Source: CAD feature listing. Evaluate the final solid. Frame: model axes, mm. Give positions to 0.01 mm unless a question says otherwise; leave off trailing zeros. Order: outer loops, then holes, each group sorted by start corner. A loop starts at its lowest first (then second) coordinate and runs counter-clockwise, first axis right, second up. Notation, with made-up numbers: (-1.75, 64) -> (15.25, 64) arc R23 ccw to (15.25, 102) -> close; hole circle Ø10 at (86, 57.5). An arc over 180 degrees is marked (long way). Use CSV: the item, a comma, the result in double quotes.
Autodesk Fusion 360 part; units mm, degrees
sketch "スケッチ1" plane through (0, 0, 0) normal (0, 1, 0) x (1, 0, 0)
  line L0 (30, 20) -> (-30, 20)
  line L1 (-30, 20) -> (-30, -20)
  line L2 (-30, -20) -> (30, -20)
  line L3 (30, -20) -> (30, 20)
  line L4 (30, 20) -> (-30, -20) construction
  line L5 (-30, 20) -> (30, -20) construction
  line L6 (-20, 0) -> (20, 0)
  dimension "d1" = 60
  dimension "d2" = 40
  dimension "d3" = 40
extrude "押し出し1" add sketch "スケッチ1" along normal blind 10
hole "穴1" at (-20, 0, 0) at (20, 0, 0) direction (0, 1, 0) diameter 3 depth 12 tip angle 118
thread "ねじ1"
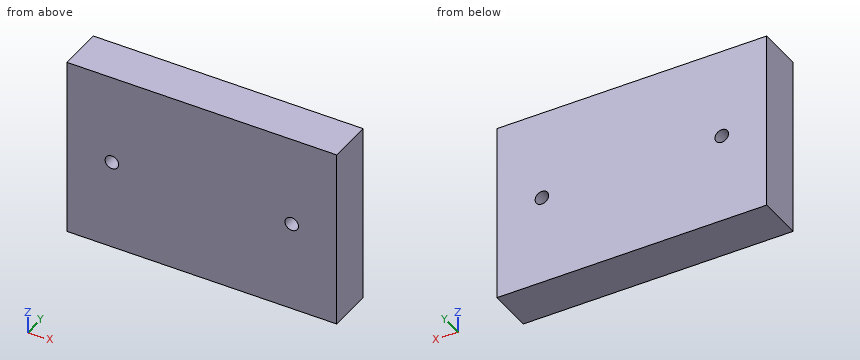
1. Section query A-A on z = 0. Return loops of the section in (x, y), plus the area to 3 significant figures.
Answer below:
outline,"(-30, 0) -> (-21.5, 0) -> (-21.5, 10) -> (-30, 10) -> close; (-18.5, 0) -> (18.5, 0) -> (18.5, 10) -> (-18.5, 10) -> close; (21.5, 0) -> (30, 0) -> (30, 10) -> (21.5, 10) -> close"
area,"540 mm²"
2. Ray query, line 1 along X through (y, z) = (6.75, 0); line 2 along Z through (x, y) = (-20, 5); line 3 along X through (y, z) = (6, 0.5). Return the intervals inside material, ascending.
Answer below:
line 1,"x = -30 to -21.5, -18.5 to 18.5, 21.5 to 30"
line 2,"z = -20 to -1.5, 1.5 to 20"
line 3,"x = -30 to -21.41, -18.59 to 18.59, 21.41 to 30"
3. Section query B-B on x = -20. Return loops of the section in (y, z).
Answer below:
outline,"(0, -20) -> (10, -20) -> (10, -1.5) -> (0, -1.5) -> close; (0, 1.5) -> (10, 1.5) -> (10, 20) -> (0, 20) -> close"
